For this review, take the finished solid that the model builds, in its own axes (mm). A direction names the side the tool comes from. Give positions to 0.01 mm unless a question says otherwise; leave off trailing zeros. Order: outer loops, then holes, each group sorted by start corner. A loop starts at its lowest first (then second) coordinate and runs counter-clockwise, first axis right, second up.
Item 1: Consider section C-C (y = -15). Give the boundary of the cut face in (x, z), plus the area to 3 significant figures.
Item 2: For P1, Ø4, axis at x = -20.5, z = 25.5, coming from the -Y side; P2, Ø12, axis at x = -23.5, y = -6, coming from the +Z side; P3, Ø4, axis at y = -5, z = 12.5, coming from the -X side; P4, Ø4, axis at y = 0.5, z = 28, coming from the -X side, all flat-tipped, find the tip position at first contact; note any pin that passes through.
Item 3: For probe 1 along Y at (x, z) = (0, 0.85); probe 2 along Y at (x, z) = (-8, 0.75); probe 3 along X at (y, z) = (1, 9), list the stretches that pass through material, from the lowest coordinate up.
Item 4: Machinability: for faces 4 (the flat face through (0, 0, 0)), 5 (the flat face through (-0.4, -6.7, 3)), 6 (the flat face through (-13.525, -11.888, 1.479)), which of the approach directions +Z, -Z, +X, -X, +Y, -Y give a long, thin tool a straight path to every point of the face, cutting with its end or side? Answer none if there is none.
Item 5: Consider section D-D (z = 28.5). Give the boundary of the cut face in (x, y).
Item 6: Consider section B-B (y = -8). Give the boundary of the cut face in (x, z), plus the area to 3 significant figures.
Item 7: Consider section A-A (x = 0). Give the boundary of the cut face in (y, z).
Item 8: The part is to be moulded in two halves that separate along X. For faces 1 (the cylindrical face through (-28, -21, 23)), 2 (the flat face through (15.4, -28.4, 46)), 3 (the cylindrical face through (-6.94, -31.24, 24.2)), say which applies: released by +X, released by -X, zero draft, split by the parting line, or undercut.
```python
from build123d import *

# Parameters (mm, degrees)
SKETCH_R           = 35
PAD_DEPTH          = 3
SKETCH001_R        = 1.2
HOLE_DEPTH         = 201.081792
POLARPATTERN_COUNT = 4
SKETCH002_R        = 35
SKETCH002_R_2      = 32
PAD001_DEPTH       = 43


with BuildPart() as part:
    # Sketch → Pad (new body)
    with BuildSketch(Plane.XY):
        Circle(SKETCH_R)
        with BuildLine():
            ThreePointArc((9.27573, -5.912769), (0, 11), (-9.27573, -5.912769))
            Line((-17.657478, -17.697838), (-9.27573, -5.912769))
            ThreePointArc((17.657478, -17.697838), (0, 25), (-17.657478, -17.697838))
            Line((9.27573, -5.912769), (17.657478, -17.697838))
        make_face(mode=Mode.SUBTRACT)
    extrude(amount=PAD_DEPTH)

    # Sketch001 (on Face7 of Pad) → Hole (cut, through all)
    with BuildSketch(Plane.XY.offset(3)):
        with Locations((0, 8)):
            Circle(SKETCH001_R)
    hole = extrude(amount=-HOLE_DEPTH, mode=Mode.SUBTRACT)

    # PolarPattern: Hole ×4 about axis
    polarpattern_axis = Axis((0, 0, 0), (0, 0, 1))
    for i in range(1, POLARPATTERN_COUNT):
        add(hole.rotate(polarpattern_axis, i * 360 / POLARPATTERN_COUNT), mode=Mode.SUBTRACT)

    # Sketch002 (on Face3 of PolarPattern) → Pad001 (join)
    with BuildSketch(Plane.XY.offset(3)):
        Circle(SKETCH002_R)
        Circle(SKETCH002_R_2, mode=Mode.SUBTRACT)
    extrude(amount=PAD001_DEPTH)


solid = part.part
```
Resolved:
1. outline: (-31.62, 0) - (-20, 0) - (-20, 3) - (-28.27, 3) - (-28.27, 46) - (-31.62, 46) - close; (-15.74, 0) - (15.74, 0) - (15.74, 3) - (-15.74, 3) - close; (20, 0) - (31.62, 0) - (31.62, 46) - (28.27, 46) - (28.27, 3) - (20, 3) - close
1. area: 453 mm2
2. P1: stops at y = -29.71
2. P2: stops at z = 3
2. P3: stops at x = -34.87
2. P4: stops at x = -35
3. probe 1: y = -35 to -9.2, -6.8 to 6.8, 9.2 to 11, 25 to 35
3. probe 2: y = -34.07 to -1.2, 1.2 to 7.55, 23.69 to 34.07
3. probe 3: x = -34.99 to -31.98, 31.98 to 34.99
4. face 4: -Z, +X, -X, +Y, -Y
4. face 5: +Z
4. face 6: +Z, -Z
5. outline: circle Ø70 at (0, 0); hole circle Ø64 at (0, 0)
6. outline: (-34.07, 0) - (-23.69, 0) - (-23.69, 3) - (-30.98, 3) - (-30.98, 46) - (-34.07, 46) - close; (-10.76, 0) - (-1.2, 0) - (-1.2, 3) - (-10.76, 3) - close; (1.2, 0) - (10.76, 0) - (10.76, 3) - (1.2, 3) - close; (23.69, 0) - (34.07, 0) - (34.07, 46) - (30.98, 46) - (30.98, 3) - (23.69, 3) - close
6. area: 385 mm2
7. outline: (-35, 0) - (-9.2, 0) - (-9.2, 3) - (-32, 3) - (-32, 46) - (-35, 46) - close; (-6.8, 0) - (6.8, 0) - (6.8, 3) - (-6.8, 3) - close; (9.2, 0) - (11, 0) - (11, 3) - (9.2, 3) - close; (25, 0) - (35, 0) - (35, 46) - (32, 46) - (32, 3) - (25, 3) - close
8. face 1: split by the parting line
8. face 2: zero draft
8. face 3: undercut
